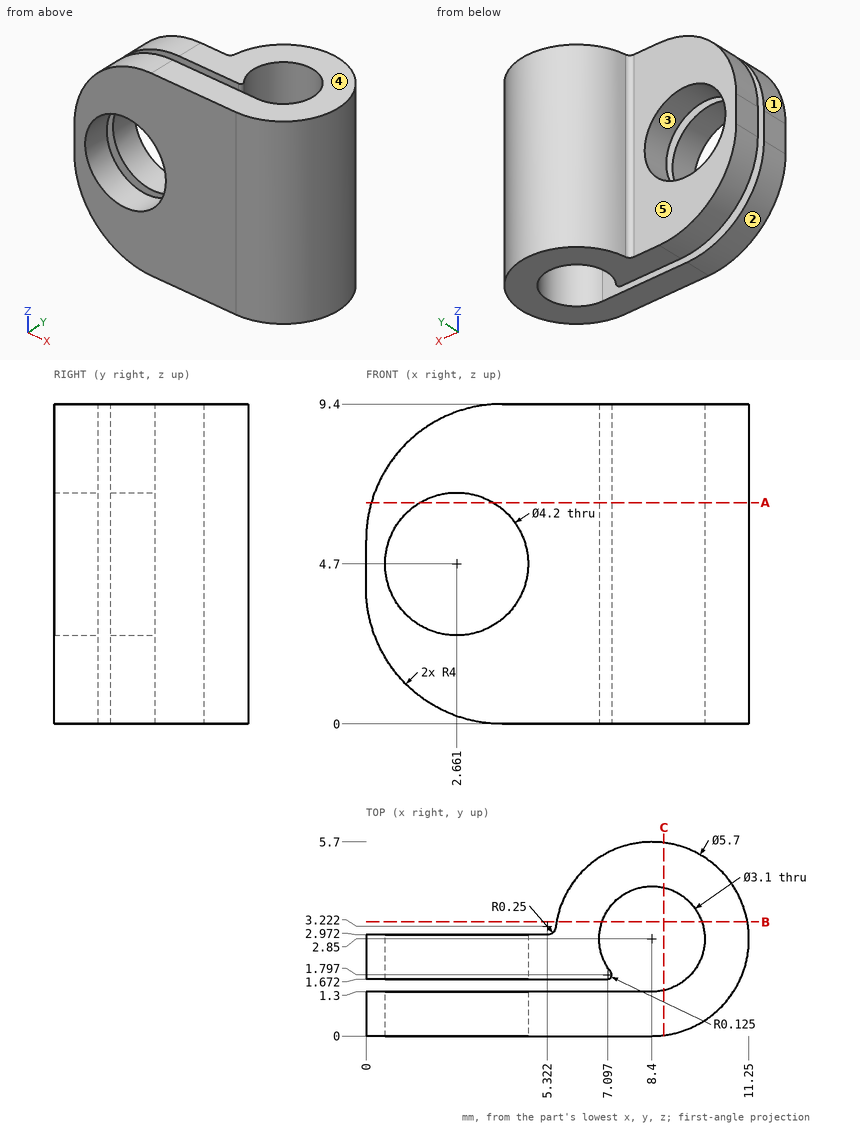
Check sheet for the drawn part. Datum: minimum x, y, z corner. Units: mm. A direction names the side the tool comes from. Round coordinates to 2 decimals unless told otherwise and drop trailing zeros. Loops run counter-clockwise (first coordinate to the right, second up) from the corner with the lowest first, then second, coordinate; pieces in that order, holes last. Notation, with made-up numbers: (49, 74.25) - (86, 74.25) arc R5 ccw to (86, 81.25) - close; hole circle Ø10 at (16.5, -11.5). An arc over 180 degrees is marked (long way). Write item = value, one per line. Start each with the question number.
1. Mould release check, pull along Z, two halves, no side actions. Record for the marked faces 1, 2 and 3: released by +Z, released by -Z, zero draft, split by the parting line, or undercut.
2. Thickness scan on line 1 (Y direction, x = 1.25, z = 6.75); line 2 (Y direction, x = 9.75, z = 6.5) (1 decimal); line 3 (Z direction, x = 1.5, y = 1). Record the ranges inside material, lowest first.
3. Section check A-A on z = 6.5. Give the number of separate pieces and of enclosed holes in the cut face, then the cut area to 3 significant figures.
4. Depth check by flat-ended pin: pin 1 (2 mm diameter, centred on y = 1, z = 2.5, fed in from -X); pin 2 (1.5 mm diameter, centred on y = 5, z = 4, fed in from +X). Enter the tip coordinate at first touch or a pass-through.
5. Section check B-B on y = 3.35. Enter the section's corners in (x, z) (1 decimal).
6. Section check C-C on x = 8.75. Enter the section's corners in (y, z), then the cut area to 3 significant figures.
7. Set-up check for the marked faces 4 and 5: record each of +Z, -Z, +X, -X, +Y, -Y from which the full face is reachable in a straight line by a thin tool's end or side.
Working result:
q1.face_1 = released by +Z
q1.face_2 = released by -Z
q1.face_3 = undercut
q2.line_1 = 0 to 1.3, 1.67 to 2.97
q2.line_2 = 0.3 to 2.1, 3.6 to 5.4
q2.line_3 = 0.88 to 2.95, 6.45 to 8.52
q3.separate_pieces = 3
q3.enclosed_holes = 0
q3.area = 27.3 mm^2
q4.pin_1 = 0.03
q4.pin_2 = 10.88
q5.outline = (5.6, 0) - (6.9, 0) - (6.9, 9.4) - (5.6, 9.4) - close; (9.9, 0) - (11.2, 0) - (11.2, 9.4) - (9.9, 9.4) - close
q6.outline = (0.02, 0) - (1.34, 0) - (1.34, 9.4) - (0.02, 9.4) - close; (4.36, 0) - (5.68, 0) - (5.68, 9.4) - (4.36, 9.4) - close
q6.area = 24.8 mm^2
q7.face_4 = +Z, +X, -X, +Y, -Y
q7.face_5 = +Z, -Z, -X, +Y
